Design review of the part shown in the three views and the two pictorial views. Dimensions are in mm from the part's minimum x, y and z. A direction names the side the tool comes from. Round coordinates to 2 decimals unless told otherwise and drop trailing zeros. Write each loop counter-clockwise with the first axis right and the second up, starting at its lowest first coordinate (ties: lowest second). Pieces come first, ordered by that corner, then holes. Notation, with made-up numbers: (54, -2.5) - (97, -2.5) arc R34 cw to (97, 33.5) - close; hole circle Ø4 at (26, -19.75). An arc over 180 degrees is marked (long way). Use one line per item in the form item = value.
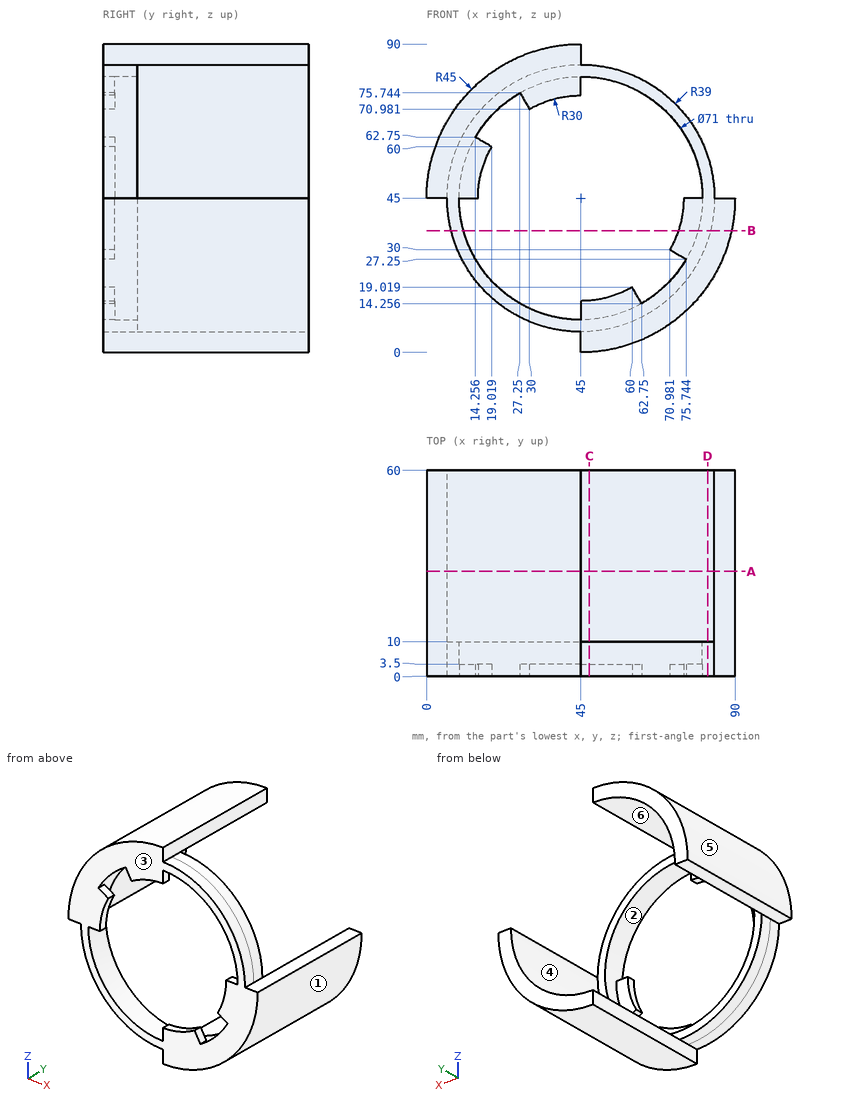
Q1. Draft analysis for pull direction X (two halves, no side actions). For the marked faces 1, 2 and 3, state which applies: released by +X, released by -X, zero draft, split by the parting line, or undercut.
Calculated:
face_1 = released by +X
face_2 = undercut
face_3 = zero draft
Q2. We need section B-B on z = 35.5. Write out the cut boundary in (x, y) (1 decimal), then the cut area to 3 significant figures.
Calculated:
outline = (7.2, 0) - (10.8, 0) - (10.8, 10) - (7.2, 10) - close; (73.5, 0) - (89, 0) - (89, 60) - (82.8, 60) - (82.8, 10) - (79.2, 10) - (79.2, 3.5) - (73.5, 3.5) - close
area = 462 mm2
Q3. We need section D-D on x = 82. Write out the cut boundary in (y, z), then the cut area to 3 significant figures.
Calculated:
outline = (0, 19.39) - (60, 19.39) - (60, 32.67) - (10, 32.67) - (10, 57.33) - (0, 57.33) - close
area = 1,040 mm2
Q4. Machinability: for the marked faces 4, 5 and 6, which of the approach directions +Z, -Z, +X, -X, +Y, -Y give a long, thin tool a straight path to every point of the face, cutting with its end or side? Answer none if there is none.
Calculated:
face_4 = +Z, -X, +Y
face_5 = +Z, -X, +Y, -Y
face_6 = -Z, +X, +Y
Q5. For P1, Ø1, axis at y = 2, z = 13, coming from the -X side (1 decimal); P2, Ø4, axis at x = 61.5, y = 34, coming from the +Z side; P3, Ø1.8, axis at x = 87, y = 28.5, coming from the +Z side; P4, Ø23.5, axis at x = 37, z = 29.5, coming from the +Y side, all flat-tipped, find the tip position at first contact; note any pin that passes through.
Calculated:
P1 = 22
P2 = 10.67
P3 = 45
P4 = through
Q6. We need section C-C on x = 47.5. Write out the cut boundary in (y, z), then the cut area to 3 significant figures.
Calculated:
outline = (0, 0.07) - (60, 0.07) - (60, 6.08) - (10, 6.08) - (10, 9.59) - (3.5, 9.59) - (3.5, 15.1) - (0, 15.1) - close; (0, 80.41) - (10, 80.41) - (10, 83.92) - (0, 83.92) - close
area = 450 mm2
Q7. To check wall thickness, follow line 1 along Y through (x, z) = (40.5, 81); line 2 along X through (y, z) = (4.5, 67.5) (1 decimal); line 3 along Y through (x, z) = (40, 77). State the ranges of each line that lie inside material, in increasing order. Write a range as from..to.
Calculated:
line_1 = 0..10
line_2 = 6..17.5, 72.5..76.9
line_3 = 0..3.5
Q8. We need section A-A on y = 30.5. Write out the cut boundary in (x, z), then the cut area to 3 significant figures.
Calculated:
outline = (0, 45) - (6, 45) arc R39 cw to (45, 84) - (45, 90) arc R45 ccw to start; (45, 0) arc R45 ccw to (90, 45) - (84, 45) arc R39 cw to (45, 6) - close
area = 792 mm2
